For this review, use the dimensioned drawing (mm, ordinates from the lowest corner) and the shaded views. A direction names the side the tool comes from. Coordinates: 2 decimals unless noted, no trailing zeros. Loops run counter-clockwise (first coordinate to the right, second up) from the corner with the lowest first, then second, coordinate; pieces in that order, holes last.
1. To check wall thickness, follow probe 1 along X at (y, z) = (24.5, 4); probe 2 along Z at (x, y) = (38, 17); probe 3 along X at (y, z) = (25, 7.75) (1 decimal). State the ranges of each line that lie inside material, in increasing order.
2. Take a section at A-A, the plane z = 6. State the section outline as (x, y) points (1 decimal).
3. Clearance check with flat-ended pins moving along their axes: P1, Ø6, axis at x = 20.5, y = 22.5, coming from the -Z side; P2, Ø2, axis at y = 44.5, z = 1, coming from the +X side; P3, Ø4, axis at x = 37.5, z = 2, coming from the +Y side (1 decimal); P4, Ø2, axis at x = 39.5, z = 6, coming from the -Y side. State where each tip first meets the part, or that it passes through.
4. Machinability: for the marked faces 1 and 2, which of the approach directions +Z, -Z, +X, -X, +Y, -Y give a long, thin tool a straight path to every point of the face, cutting with its end or side? Answer none if there is none.
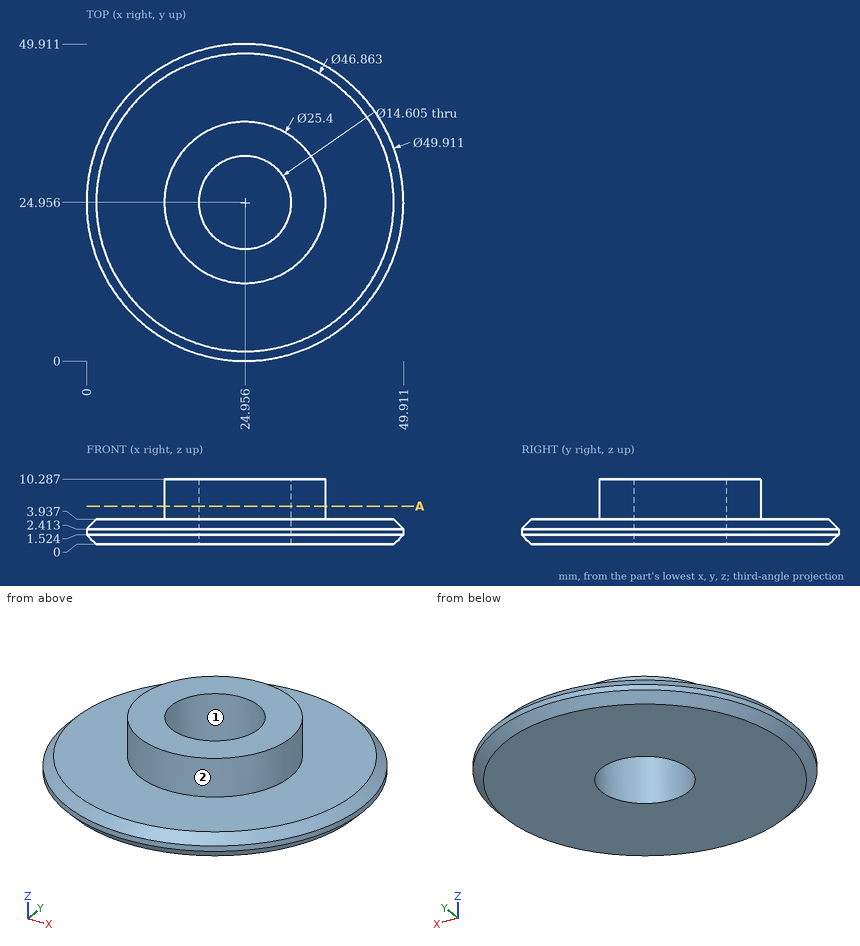
Results list:
1. probe 1: x = 12.26 to 17.67, 32.24 to 37.65
1. probe 2: z = 0 to 3.94
1. probe 3: x = 12.3 to 17.7, 32.3 to 37.7
2. outline: circle Ø25.4 at (25, 25); hole circle Ø14.6 at (25, 25)
3. P1: stops at z = 0
3. P2: stops at x = 41.49
3. P3: stops at y = 47.6
3. P4: passes through
4. face 1: +Z, -Z
4. face 2: +Z
